from build123d import *

# Parameters (mm, degrees)
SKETCH1_W           = 79
SKETCH1_H           = 8.5
SKETCH1_R           = 2.125
BOSS_EXTRUDE1_DEPTH = 2
SKETCH3_W           = 58.5
SKETCH3_H           = 7.5
BOSS_EXTRUDE2_DEPTH = 40.14
SKETCH4_W           = 58.5
SKETCH4_H           = 2
BOSS_EXTRUDE3_DEPTH = 12.5
CUT_EXTRUDE1_REACH  = 93.966
SKETCH5_R           = 2.125
FILLET1_R           = 2
FILLET2_R           = 1
FILLET3_R           = 2
FILLET4_R           = 1
FILLET5_R           = 1


with BuildPart() as part:
    # Sketch1 → Boss-Extrude1 (new body)
    with BuildSketch(Plane(origin=(0, 0, 0), x_dir=(1, 0, 0), z_dir=(0, 1, 0))):
        with Locations((-39.5, 4.25)):
            Rectangle(SKETCH1_W, SKETCH1_H)
        with Locations(Location((-74.75, 4.25, 0), (0, 0, 270))):
            Circle(SKETCH1_R, mode=Mode.SUBTRACT)
        with Locations(Location((-4.25, 4.25, 0), (0, 0, 270))):
            Circle(SKETCH1_R, mode=Mode.SUBTRACT)
    extrude(amount=BOSS_EXTRUDE1_DEPTH)

    # Sketch3 → Boss-Extrude2 (add)
    with BuildSketch(Plane(origin=(0, 2, 0), x_dir=(1, 0, 0), z_dir=(0, 1, 0))):
        with Locations((-39.5, 4.75)):
            Rectangle(SKETCH3_W, SKETCH3_H)
    extrude(amount=BOSS_EXTRUDE2_DEPTH)

    # Sketch4 → Boss-Extrude3 (add)
    with BuildSketch(Plane(origin=(0, 0, -8.5), x_dir=(-1, 0, 0), z_dir=(0, 0, -1))):
        with Locations((39.5, 41.14)):
            Rectangle(SKETCH4_W, SKETCH4_H)
    extrude(amount=BOSS_EXTRUDE3_DEPTH)

    # Sketch5 → Cut-Extrude1 (cut, up to next)
    with BuildSketch(Plane(origin=(0, 42.14, 0), x_dir=(1, 0, 0), z_dir=(0, 1, 0)), mode=Mode.PRIVATE) as cut_extrude1_sk1:
        with Locations(Location((-14.5, 16.75, 0), (0, 0, 270))):
            Circle(SKETCH5_R)
    cut_extrude1_tool1 = extrude(cut_extrude1_sk1.sketch, amount=-CUT_EXTRUDE1_REACH, mode=Mode.PRIVATE) & part.part
    # Sketch5 → Cut-Extrude1 (cut, up to next)
    with BuildSketch(Plane(origin=(0, 42.14, 0), x_dir=(1, 0, 0), z_dir=(0, 1, 0)), mode=Mode.PRIVATE) as cut_extrude1_sk2:
        with Locations(Location((-64.5, 16.75, 0), (0, 0, 270))):
            Circle(SKETCH5_R)
    cut_extrude1_tool2 = extrude(cut_extrude1_sk2.sketch, amount=-CUT_EXTRUDE1_REACH, mode=Mode.PRIVATE) & part.part
    add(cut_extrude1_tool1.solids().sort_by_distance((-14.5, 42.14, -16.75))[0], mode=Mode.SUBTRACT)
    add(cut_extrude1_tool2.solids().sort_by_distance((-64.5, 42.14, -16.75))[0], mode=Mode.SUBTRACT)

    # Fillet1
    # the kernel refuses this fillet: 2 mm, written as the material it adds along each edge
    with BuildSketch(Plane(origin=(-68.75, 40.14, -8.5), x_dir=(0, -1, 0), z_dir=(1, 0, 0))) as fillet1_piece_1:
        with BuildLine():
            CenterArc((FILLET1_R, FILLET1_R), FILLET1_R, 180, 90)
            Line((0, FILLET1_R), (-FILLET1_R * 0.02, FILLET1_R))
            Line((-FILLET1_R * 0.02, FILLET1_R), (-FILLET1_R * 0.02, -FILLET1_R * 0.02))
            Line((-FILLET1_R * 0.02, -FILLET1_R * 0.02), (FILLET1_R, -FILLET1_R * 0.02))
            Line((FILLET1_R, -FILLET1_R * 0.02), (FILLET1_R, 0))
        make_face()
    extrude(amount=58.5)
    with BuildSketch(Plane(origin=(-68.75, 2, -1), x_dir=(0, 0, 1), z_dir=(1, 0, 0))) as fillet1_piece_2:
        with BuildLine():
            CenterArc((2, -1.732050808), FILLET1_R, 120, 60)
            Line((0, -1.732050808), (-0.04, -1.732050808))
            Line((-0.04, -1.732050808), (-0.04, 0))
            Line((-0.04, 0), (0, 0.04))
            ThreePointArc((0, 0.04), (0.5, 0.04), (0.98, 0.034641016))
            Line((0.98, 0.034641016), (1, 0))
        make_face()
    extrude(amount=58.5)

    # Fillet2
    fillet2_edges = [part.edges().sort_by_distance(p)[0] for p in [
        (-79, 1, 0),
        (-79, 1, -8.5),
        (-68.75, 41.14, -21),
        (-10.25, 41.14, -21),
        (0, 1, -8.5),
        (0, 1, 0),
    ]]
    fillet(fillet2_edges, radius=FILLET2_R)

    # Fillet3
    fillet3_edges = [part.edges().sort_by_distance(p)[0] for p in [
        (-39.5, 42.14, -1),
    ]]
    fillet(fillet3_edges, radius=FILLET3_R)

    # Fillet4
    # the kernel refuses this fillet: 1 mm, written as the material it adds along each edge
    with BuildSketch(Plane(origin=(-10.25, 2, 0), x_dir=(0, 1, 0), z_dir=(0, 0, -1))) as fillet4_piece_1_section:
        with BuildLine():
            CenterArc((FILLET4_R, FILLET4_R), FILLET4_R, 180, 90)
            Line((0, FILLET4_R), (0, 0))
            Line((0, 0), (FILLET4_R, 0))
        make_face()
    fillet4_piece_1 = extrude(amount=8.5, mode=Mode.PRIVATE)
    fillet4_piece_1 = fillet4_piece_1 - Plane(origin=(-10.019982346, 3.732050808, 1), x_dir=(0, 0, 1), z_dir=(-1, 0, 0)) * Cylinder(2, 21, mode=Mode.PRIVATE)
    add(fillet4_piece_1)

    # Fillet5
    # the kernel refuses this fillet: 1 mm, written as the material it adds along each edge
    with BuildSketch(Plane(origin=(-68.75, 2, -8.5), x_dir=(-1, 0, 0), z_dir=(0, 0, 1))) as fillet5_piece_1_section:
        with BuildLine():
            CenterArc((FILLET5_R, -FILLET5_R), FILLET5_R, 90, 90)
            Line((0, -FILLET5_R), (0, 0))
            Line((0, 0), (FILLET5_R, 0))
        make_face()
    fillet5_piece_1 = extrude(amount=8.5, mode=Mode.PRIVATE)
    fillet5_piece_1 = fillet5_piece_1 - Plane(origin=(-68.980019627, 3.732050808, 1), x_dir=(0, 0, 1), z_dir=(-1, 0, 0)) * Cylinder(2, 21, mode=Mode.PRIVATE)
    add(fillet5_piece_1)


solid = part.part
Source: CAD feature listing. Evaluate the final solid. Frame: model axes, mm. A direction names the side the tool comes from. Round coordinates to 2 decimals unless told otherwise and drop trailing zeros. Loops run counter-clockwise (first coordinate to the right, second up) from the corner with the lowest first, then second, coordinate; pieces in that order, holes last. Notation, with made-up numbers: M -31,51 L 17,51 A31 ccw 17,83 Z; hole C 16,69 d11. An arc over 180 degrees is marked long. Return JSON: item names as keys, results as strings. Group by question number.
1. Section query C-C on x = -23.5. Output: boundary loops of the cut face in (y, z), and give its area (3 significant figures).
2. Section query D-D on z = -16.75. Output: boundary loops of the cut face in (x, y) (3 decimals), and give its area (3 significant figures).
3. Reachability of faces 1 (the face through (-7, 2, -4)), 2 (the face through (-40, 19, -8.5)), 3 (the face through (-72, 2, -4)), 4 (the face through (-40, 22, -1)) from +Z, -Z, +X, -X, +Y, -Y: full face, straight path, thin tool, end or side. Return the list, or none.
4. Mould query, pull axis X, two halves, no side actions, for faces 5 (the face through (-79, 1, -4)), 6 (the face through (-63.064, 41.154, -18.316)), 7 (the face through (-39.91, 39.57, -9.1)), 8 (the face through (-10.25, 22, -6)). Classes: released by +X, released by -X, zero draft, split by the parting line, or undercut.
5. Section query B-B on x = -4.25. Output: boundary loops of the cut face in (y, z) (3 decimals), and give its area (3 significant figures).
6. Pin query (flat end, axial travel): pin 1 (12 mm diameter, centred on x = -40.5, y = 34, fed in from +Z); pin 2 (2.5 mm diameter, centred on x = -4.5, z = -2.5, fed in from +Y); pin 3 (5.5 mm diameter, centred on y = 31.5, z = -10.5, fed in from +X). Return the tip coordinate at first contact, or that it passes through.
7. Section query A-A on z = -4.25. Output: boundary loops of the cut face in (x, y) (3 decimals), and give its area (3 significant figures).
8. Material intervals for line 1 along X through (y, z) = (0.55, -4.25) (3 decimals); line 2 along Z through (x, y) = (-65, 21); line 3 along Y through (x, z) = (-72, -3), sorted ascending. Write a range as from..to.
Checks:
{
 "1": {"outline": "M 0,-8.5 L 38.14,-8.5 A2 cw 40.14,-10.5 L 40.14,-21 L 42.14,-21 L 42.14,-3 A2 ccw 40.14,-1 L 3.73,-1 A2 cw 2,0 L 0,0 Z", "area": "344 mm²"},
 "2": {"outline": "M -68.75,40.14 L -66.625,40.14 L -66.625,42.14 L -68.75,42.14 Z; M -62.375,40.14 L -16.625,40.14 L -16.625,42.14 L -62.375,42.14 Z; M -12.375,40.14 L -10.25,40.14 L -10.25,42.14 L -12.375,42.14 Z", "area": "100 mm²"},
 "3": {"face 1": "+Z, -Z, +X, +Y", "face 2": "-Z, +X, -X, -Y", "face 3": "+Z, -Z, -X, +Y", "face 4": "+Z, +X, -X, +Y"},
 "4": {"face 5": "released by -X", "face 6": "undercut", "face 7": "zero draft", "face 8": "released by +X"},
 "5": {"outline": "M 0,-8.5 L 2,-8.5 L 2,-6.375 L 0,-6.375 Z; M 0,-2.125 L 2,-2.125 L 2,0 L 0,0 Z", "area": "8.50 mm²"},
 "6": {"pin 1": "stops at z = -1", "pin 2": "stops at y = 2", "pin 3": "stops at x = -10.25"},
 "7": {"outline": "M -79,0 L -76.875,0 L -76.875,2 L -79,2 Z; M -72.625,0 L -6.375,0 L -6.375,2 L -9.25,2 A1 cw -10.25,3 L -10.25,42.14 L -68.75,42.14 L -68.75,3 A1 cw -69.75,2 L -72.625,2 Z; M -2.125,0 L 0,0 L 0,2 L -2.125,2 Z", "area": "2,490 mm²"},
 "8": {"line 1": "x = -79..-76.875, -72.625..-6.375, -2.125..0", "line 2": "z = -8.5..-1", "line 3": "y = 0..2"}
}
